Geometry: final body of the model. Coordinates: model frame, mm. A direction names the side the tool comes from. Give positions to 0.01 mm unless a question says otherwise; leave off trailing zeros. Loops run counter-clockwise (first coordinate to the right, second up) from the corner with the lowest first, then second, coordinate; pieces in that order, holes last. Notation, with made-up numbers: (68.25, 11.25) - (116.25, 11.25) arc R21 ccw to (116.25, 15.25) - close; hole circle Ø7 at (28.25, -25.5). An arc over 180 degrees is marked (long way). Answer in a Markdown table with one row per item.
Autodesk Inventor part; units mm, degrees
ref_plane "YZ Plane" through (0, 0, 0) normal (1, 0, 0) x (0, 1, 0)
ref_plane "XZ Plane" through (0, 0, 0) normal (0, 1, 0) x (-1, 0, 0)
ref_plane "XY Plane" through (0, 0, 0) normal (0, 0, 1) x (1, 0, 0)
sketch "Sketch1" plane through (0, 0, 0) normal (0, 0, 1) x (1, 0, 0)
  line L0 (-35.56, 0) -> (35.56, 0)
  line L1 (0, -17.78) -> (0, 17.78)
  line L2 (-25.4, 12.7) -> (25.4, 12.7)
  line L3 (25.4, 12.7) -> (25.4, -12.7)
  line L4 (25.4, -12.7) -> (-25.4, -12.7)
  line L5 (-25.4, -12.7) -> (-25.4, 12.7)
  line L6 (22.225, 9.525) -> (-22.225, 9.525)
  line L7 (-22.225, 9.525) -> (-22.225, -9.525)
  line L8 (-22.225, -9.525) -> (22.225, -9.525)
  line L9 (22.225, -9.525) -> (22.225, 9.525)
  point P0 (0, 0)
  point P1 (-25.4, 0)
  point P2 (0, 12.7)
  dimension "d0" = 25.4
  dimension "d1" = 3.175
  dimension "d7" = 50.8
extrude "Extrusion1" add sketch "Sketch1" along normal mid plane 254 contours L5 L2 L1 L6 L7 L0 | L0 L7 L8 L1 L4 L5 | L1 L8 L9 L0 L3 L4 | L2 L3 L0 L9 L6 L1
sketch "Sketch3" plane through (-25.4, 12.7, 127) normal (0, 1, 0) x (1, 0, 0)
  line L0 (0, 0) -> (50.8, 0)
  circle A0 centre (25.4, 78.74) radius 15.9131
  point P0 (25.4, 127)
  dimension "d8" = 31.8262
  dimension "d9" = 78.74
extrude "Extrusion3" cut sketch "Sketch3" against normal up to surface (3.175 mm away)
sketch "Sketch4" plane through (-25.4, -12.7, 127) normal (0, -1, 0) x (1, 0, 0)
  line L0 (50.8, 0) -> (0, 0)
  circle A0 centre (25.4, -78.74) radius 7.9375
  point P0 (25.4, -127)
  dimension "d12" = 15.875
  dimension "d13" = 78.74
extrude "Extrusion4" cut sketch "Sketch4" against normal up to surface (3.175 mm away)
sketch "Sketch5" plane through (-25.4, 12.7, 127) normal (0, 1, 0) x (1, 0, 0)
  circle A0 centre (25.4, 78.74) radius 15.9131
  point P0 (25.4, 127)
  point P1 (25.4, 104.14)
  point P2 (25.4, 53.34)
  dimension "d16" = 25.4
  dimension "d17" = 25.4
hole "Hole1" at (0, 12.7, 22.86) at (0, 12.7, 73.66) direction (0, -1, 0) diameter 6.7564 end through all
properties part number "tubing_template_0.125" material "Aluminum-6061"
Q1. Reachability of faces 1 (the cylindrical face through (-2.072, 11.135, 32.482)), 2 (the cylindrical face through (1.294, 11.09, 76.781)), 3 (the flat face through (22.225, 0, -2)) from +Z, -Z, +X, -X, +Y, -Y: full face, straight path, thin tool, end or side. Return the list, or none.
Check values:
| item | result |
|---|---|
| face 1 | +Y |
| face 2 | +Y, -Y |
| face 3 | +Z, -Z |
Q2. Cut plane C-C (z = -10.5). Output: boundary loops of the cut face in (x, y) (3 decimals), and give its area (3 significant figures).
Check values:
| item | result |
|---|---|
| outline | (-25.4, -12.7) - (25.4, -12.7) - (25.4, 12.7) - (-25.4, 12.7) - close; hole (-22.225, -9.525) - (22.225, -9.525) - (22.225, 9.525) - (-22.225, 9.525) - close |
| area | 444 mm² |
Q3. Material intervals for line 1 along Z through (x, y) = (0, -11.6); line 2 along Z through (x, y) = (0, 10.5); line 3 along Y through (x, z) = (-19, -80) (3 decimals), sorted ascending.
Check values:
| item | result |
|---|---|
| line 1 | -127 to 19.48, 26.24 to 40.32, 56.2 to 70.28, 77.04 to 127 |
| line 2 | -127 to 19.48, 26.24 to 32.35, 64.17 to 70.28, 77.04 to 127 |
| line 3 | -12.7 to -9.525, 9.525 to 12.7 |
Q4. Cut plane B-B (z = 48.26). Output: boundary loops of the cut face in (x, y) (1 decimal), and give its area (3 significant figures).
Check values:
| item | result |
|---|---|
| outline | (-25.4, -12.7) - (-7.9, -12.7) - (-7.9, -9.5) - (-22.2, -9.5) - (-22.2, 9.5) - (-15.9, 9.5) - (-15.9, 12.7) - (-25.4, 12.7) - close; (7.9, -12.7) - (25.4, -12.7) - (25.4, 12.7) - (15.9, 12.7) - (15.9, 9.5) - (22.2, 9.5) - (22.2, -9.5) - (7.9, -9.5) - close |
| area | 292 mm² |
Q5. Draft query along Y for faces 4 (the flat face through (-22.225, 0, -2)), 5 (the flat face through (0, 9.525, -2)), 6 (the cylindrical face through (1.294, -11.135, 76.781)), 7 (the flat face through (0, 12.7, -2)). Return one class per face: pulls with the +Y half, pulls with the -Y half, needs draft (parallel to the pull), parting line crosses it, or undercut.
Check values:
| item | result |
|---|---|
| face 4 | undercut |
| face 5 | undercut |
| face 6 | needs draft |
| face 7 | pulls with the +Y half |
Q6. Cut plane A-A (y = -0.75). Output: boundary loops of the cut face in (x, z) (3 decimals).
Check values:
| item | result |
|---|---|
| outline | (-25.4, -127) - (-22.225, -127) - (-22.225, 127) - (-25.4, 127) - close; (22.225, -127) - (25.4, -127) - (25.4, 127) - (22.225, 127) - close |
Q7. Cut plane D-D (x = 0). Give the number of separate pieces and of enclosed holes in the cut face, and give its area (3 significant figures).
Check values:
| item | result |
|---|---|
| separate pieces | 8 |
| enclosed holes | 0 |
| area | 1,380 mm² |
Q8. First-contact query: pin 1 (12.5 mm diameter, centred on x = 0, z = 48.26, fed in from -Y); pin 2 (6 mm diameter, centred on x = 1, z = 36.5, fed in from +Y) (3 decimals). Flat tips, straight axial feed; report the tip coordinate or a pass-through.
Check values:
| item | result |
|---|---|
| pin 1 | through |
| pin 2 | y = -9.525 |
